CAD build for the part. Positions are in the model's coordinates, mm. Face numbers are marked on the shaded views. A direction names the side the tool comes from. Round coordinates to 2 decimals unless told otherwise and drop trailing zeros. Write each loop counter-clockwise with the first axis right and the second up, starting at its lowest first coordinate (ties: lowest second). Pieces come first, ordered by that corner, then holes. Notation, with made-up numbers: (34.5, 7.5) - (66.5, 7.5) arc R24 ccw to (66.5, 21.5) - close; hole circle Ø11 at (-6.5, 41.5). An arc over 180 degrees is marked (long way). Answer in a Markdown table with one row per item.
```python
from build123d import *

# Parameters (mm, degrees)
F0_W      = 1000
F0_H      = 500
F1_DEPTH  = 25
F2_W      = 400
F2_H      = 350
F3_DEPTH  = 25
F4_W      = 450
F4_H      = 25
F5_DEPTH  = 165
F6_W      = 450
F6_H      = 25
F7_DEPTH  = 100
F9_DEPTH  = 25
F10_W     = 450
F10_H     = 320.7023542165
F11_DEPTH = 21.4373231428
F12_R     = 10


# Not quite as in the source:
# - a pattern or mirror of a feature is missing from the dataset's text; its kind, count and spacing are read off the source's solid


with BuildPart() as f1:
    # F0 (on Top) → F1 (new body)
    with BuildSketch(Plane.XY):
        Rectangle(F0_W, F0_H)
    extrude(amount=F1_DEPTH)

    # F2 (on face) → F3 (cut, through all)
    with BuildSketch(Plane.XY.offset(25)):
        with Locations((0, -15)):
            Rectangle(F2_W, F2_H)
    extrude(amount=-F3_DEPTH, mode=Mode.SUBTRACT)

    # F4 (on face) → F5 (join)
    with BuildSketch(Plane(origin=(0, 0, 0), x_dir=(1, 0, 0), z_dir=(0, 0, -1))):
        with Locations((0, -172.5)):
            Rectangle(F4_W, F4_H)
    extrude(amount=F5_DEPTH)

    # F6 (on face) → F7 (join)
    with BuildSketch(Plane.XZ.offset(-160)):
        with Locations((0, -152.5)):
            Rectangle(F6_W, F6_H)
    extrude(amount=F7_DEPTH)

    # F8 (on face) → F9 (join)
    with BuildSketch(Plane(origin=(-225, 0, 0), x_dir=(0, -1, 0), z_dir=(-1, 0, 0))):
        Polygon((215, 0), (-185, 0), (-185, -165), (-60, -165), align=None)
    f9 = extrude(amount=-F9_DEPTH)

    # F9_copies: F9 across plane
    add(f9.mirror(Plane(origin=(0, 0, 0), x_dir=(0, 0, 1), z_dir=(1, 0, 0))))

    # F10 (on face) → F11 (join, through all)
    with BuildSketch(Plane(origin=(0, -56.9117647059, -94.8529411765), x_dir=(1, 0, 0), z_dir=(0, -0.5144957554, -0.8574929257))):
        with Locations((0, 24.00980192)):
            Rectangle(F10_W, F10_H)
    extrude(amount=-F11_DEPTH)

    # F12
    f12_edges = [f1.edges().sort_by_distance(p)[0] for p in [
        (0, 160, -140),
        (-200, 110, -140),
        (-200, 160, -57.5),
        (0, 60, -140),
        (-200, -65, -65),
        (-200, -190, 17.5),
        (200, -190, 17.5),
        (0, -190, 10),
        (200, 160, -57.5),
        (200, 110, -140),
        (200, -65, -65),
    ]]
    fillet(f12_edges, radius=F12_R)


solid = f1.part
```
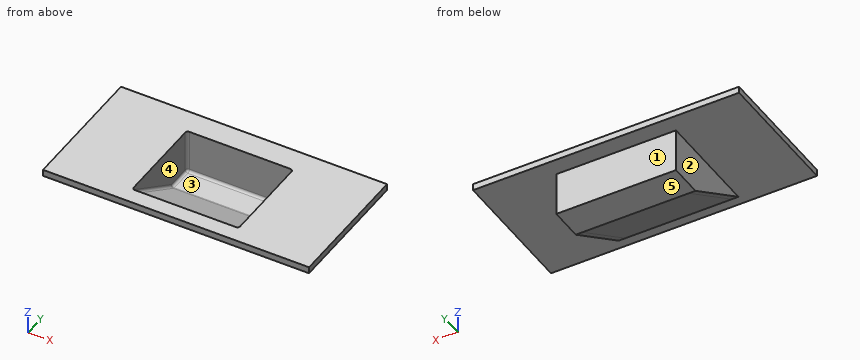
Q1. Saw through at A-A on x = 73.5. List the corners of the cut face in (y, z).
Computed:
| item | result |
|---|---|
| outline | (-250, 0) - (-215, 0) - (60, -165) - (185, -165) - (185, 0) - (250, 0) - (250, 25) - (160, 25) - (160, -130) arc R10 cw to (150, -140) - (62.77, -140) arc R10 cw to (57.62, -138.57) - (-185.14, 7.09) arc R10 cw to (-190, 15.66) - (-190, 25) - (-250, 25) - close |
Q2. 3-axis set-ups, long thin cutter, end or side, ignore diameter. For the marked faces 4 and 5: which of +Z, -Z, +X, -X, +Y, -Y reach the whole face in a straight line?
Computed:
| item | result |
|---|---|
| face 4 | +Z |
| face 5 | -Z, +X, -X, +Y, -Y |
Q3. Flat gauge pins, fed straight in: pin 1 (3 mm diameter, centred on y = 94.5, z = -118.5, fed in from +X); pin 2 (3 mm diameter, centred on x = -73, z = -10.5, fed in from -Y); pin 3 (5 mm diameter, centred on x = 169, z = -114, fed in from -Y). Where does each tip first touch, or does it go through?
Computed:
| item | result |
|---|---|
| pin 1 | stops at x = 225 |
| pin 2 | stops at y = -200 |
| pin 3 | stops at y = -29.17 |
Q4. Drill centre lines: line 1 (X direction, y = -96, z = 6); line 2 (X direction, y = 85, z = -77); line 3 (Y direction, x = 167, z = 15). Where is each one in solid material? Low to high.
Computed:
| item | result |
|---|---|
| line 1 | x = -500 to -200, 200 to 500 |
| line 2 | x = -225 to -200, 200 to 225 |
| line 3 | y = -250 to -189.98, 160 to 250 |
Q5. Saw through at D-D on y = 212. List the corners of the cut face in (x, z).
Computed:
| item | result |
|---|---|
| outline | (-500, 0) - (500, 0) - (500, 25) - (-500, 25) - close |
Q6. Saw through at C-C on x = -344. List the corners of the cut face in (y, z), then the cut area to 3 significant figures.
Computed:
| item | result |
|---|---|
| outline | (-250, 0) - (250, 0) - (250, 25) - (-250, 25) - close |
| area | 12,500 mm2 |
Q7. Pull direction Y, two halves, no side cores. Call the marked faces 1, 2 and 3: released by +Y, released by -Y, zero draft, split by the parting line, or undercut.
Computed:
| item | result |
|---|---|
| face 1 | released by +Y |
| face 2 | zero draft |
| face 3 | undercut |
Q8. Saw through at B-B on y = 97.5. List the corners of the cut face in (x, z), then the cut area to 3 significant figures.
Computed:
| item | result |
|---|---|
| outline | (-500, 0) - (-225, 0) - (-225, -165) - (225, -165) - (225, 0) - (500, 0) - (500, 25) - (200, 25) - (200, -130) arc R10 cw to (190, -140) - (-190, -140) arc R10 cw to (-200, -130) - (-200, 25) - (-500, 25) - close |
| area | 33,300 mm2 |
